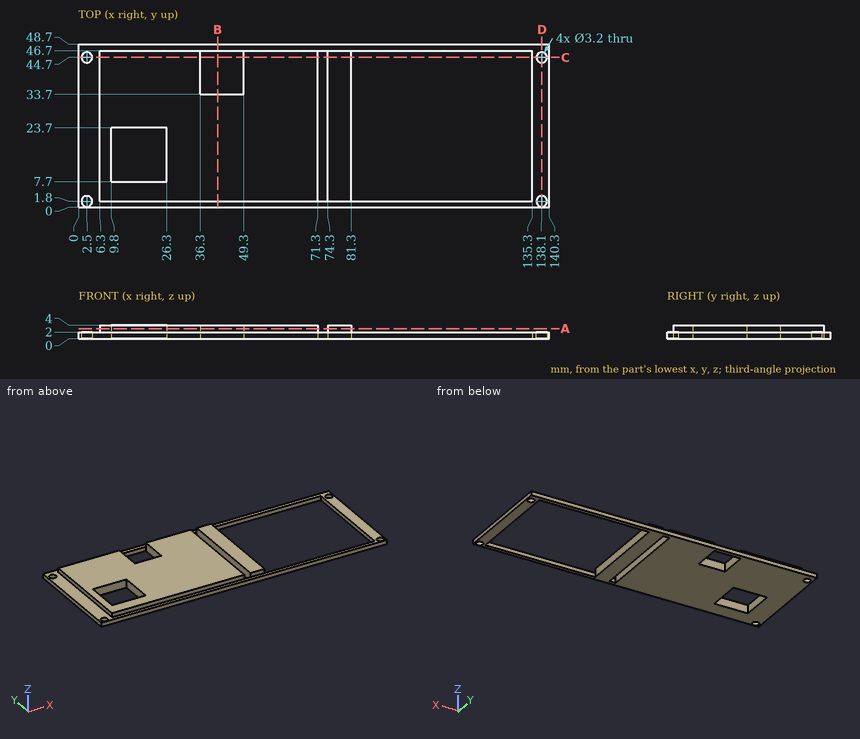
Job drawing, mm, ordinate dimensions from the low corner. One solid piece. Round coordinates to 2 decimals unless told otherwise and drop trailing zeros. Loops run counter-clockwise (first coordinate to the right, second up) from the corner with the lowest first, then second, coordinate; pieces in that order, holes last. Notation, with made-up numbers: (-25.5, -29.5) -> (9.5, -29.5) arc R8 cw to (9.5, -17.5) -> close; hole circle Ø2 at (78.25, 89.5). An arc over 180 degrees is marked (long way). Use CSV: the item, a comma, the result in double quotes. Start each with the question number.
Q1. Flat gauge pins, fed straight in: pin 1 Ø1.2 at (y, z) = (16.5, 3) entering from -X; pin 2 Ø2.5 at (x, y) = (2.5, 1.8) entering from +Z; pin 3 Ø1 at (x, z) = (76.5, 3) entering from -Y. Where does each tip first touch, or does it go through?
Q2. Saw through at D-D on x = 138.1. Give the cut face in (y, z), and give its area (3 significant figures).
Q3. Saw through at B-B on x = 41.5. Give the cut face in (y, z), and give its area (3 significant figures).
Q4. Saw through at A-A on z = 3. Give the cut face in (x, y).
Q5. Drill centre lines: L1, parallel to X at y = 40, z = 1.3; L2, parallel to Y at x = 138.1, z = 1.55; L3, parallel to X at y = 45.5, z = 2.45. Where is each one in solid material? Low to high.
Q6. Saw through at C-C on y = 44.7. Give the cut face in (x, z).
Solutions:
1,pin 1,"stops at x = 6.3"
1,pin 2,"passes through"
1,pin 3,"stops at y = 1.8"
2,outline,"(0, 0) -> (0.2, 0) -> (0.2, 2) -> (0, 2) -> close; (3.4, 0) -> (43.1, 0) -> (43.1, 2) -> (3.4, 2) -> close; (46.3, 0) -> (48.7, 0) -> (48.7, 2) -> (46.3, 2) -> close"
2,area,"84.6 mm^2"
3,outline,"(0, 0) -> (33.7, 0) -> (33.7, 4) -> (1.8, 4) -> (1.8, 2) -> (0, 2) -> close; (46.7, 0) -> (48.7, 0) -> (48.7, 2) -> (46.7, 2) -> close"
3,area,"135 mm^2"
4,outline,"(6.3, 1.8) -> (71.3, 1.8) -> (71.3, 46.7) -> (49.3, 46.7) -> (49.3, 33.7) -> (36.3, 33.7) -> (36.3, 46.7) -> (6.3, 46.7) -> close; (74.3, 1.8) -> (81.3, 1.8) -> (81.3, 46.7) -> (74.3, 46.7) -> close; hole (9.8, 7.7) -> (26.3, 7.7) -> (26.3, 23.7) -> (9.8, 23.7) -> close"
5,L1,"x = 0 to 36.3, 49.3 to 71.3, 74.3 to 81.3, 135.3 to 140.3"
5,L2,"y = 0 to 0.2, 3.4 to 43.1, 46.3 to 48.7"
5,L3,"x = 6.3 to 36.3, 49.3 to 71.3, 74.3 to 81.3"
6,outline,"(0, 0) -> (0.9, 0) -> (0.9, 2) -> (0, 2) -> close; (4.1, 0) -> (36.3, 0) -> (36.3, 4) -> (6.3, 4) -> (6.3, 2) -> (4.1, 2) -> close; (49.3, 0) -> (71.3, 0) -> (71.3, 4) -> (49.3, 4) -> close; (74.3, 0) -> (81.3, 0) -> (81.3, 4) -> (74.3, 4) -> close; (135.3, 0) -> (136.5, 0) -> (136.5, 2) -> (135.3, 2) -> close; (139.7, 0) -> (140.3, 0) -> (140.3, 2) -> (139.7, 2) -> close"
